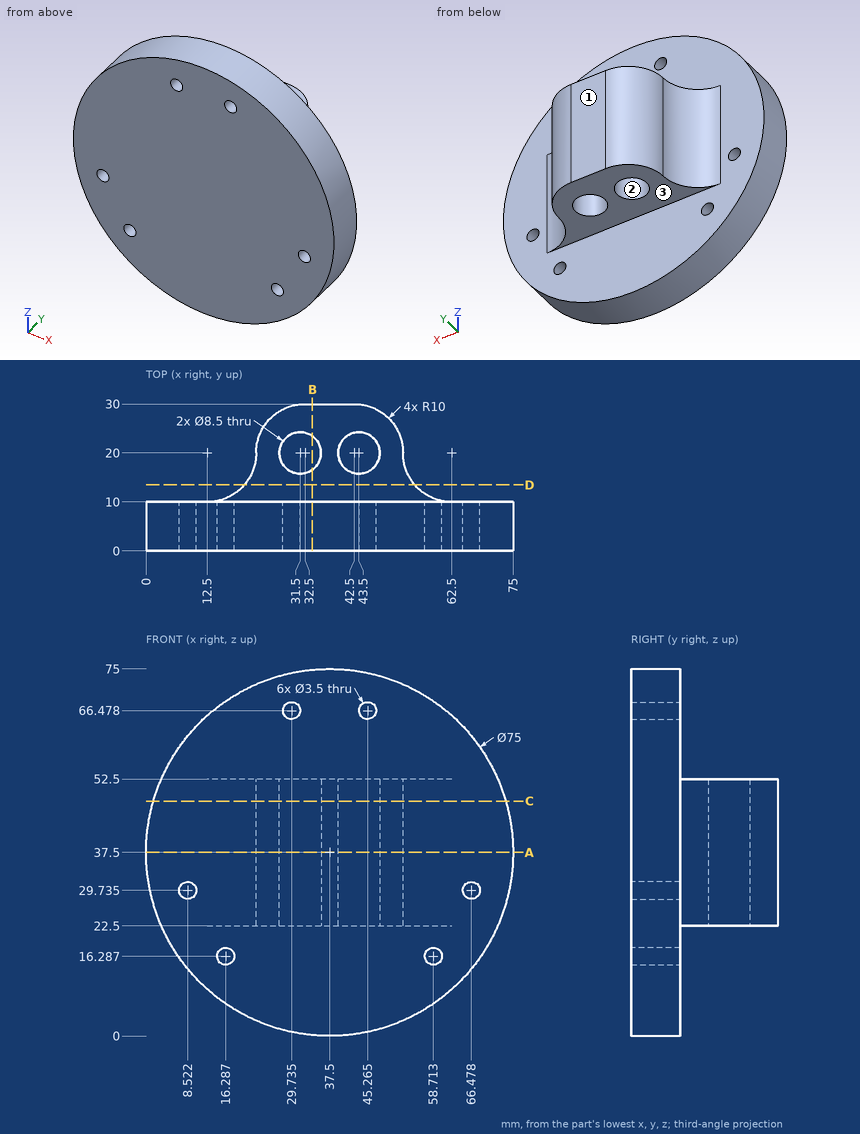
Design review of the part shown in the three views and the two pictorial views. Dimensions are in mm from the part's minimum x, y and z. Give positions to 0.01 mm unless a question says otherwise; leave off trailing zeros. Write each loop counter-clockwise with the first axis right and the second up, starting at its lowest first coordinate (ties: lowest second). Pieces come first, ordered by that corner, then holes. Notation, with made-up numbers: M 10.25,31 L 42.25,31 A28 cw 42.25,50 Z; hole C 27,82.25 d6. An arc over 180 degrees is marked long. Answer in a Markdown table with one row per item.
Item 1: Add section B-B on x = 34. Give the boundary of the cut face in (y, z).
Check sheet entries:
| item | result |
|---|---|
| outline | M 0,0.16 L 10,0.16 L 10,22.5 L 16.56,22.5 L 16.56,52.5 L 10,52.5 L 10,74.84 L 0,74.84 Z; M 23.44,22.5 L 30,22.5 L 30,52.5 L 23.44,52.5 Z |
Item 2: Add section D-D on y = 13.5. Give the boundary of the cut face in (x, z), plus the area to 3 significant figures.
Check sheet entries:
| item | result |
|---|---|
| outline | M 20.1,22.5 L 54.9,22.5 L 54.9,52.5 L 20.1,52.5 Z |
| area | 1,040 mm2 |
Item 3: Add section A-A on z = 37.5. Give the boundary of the cut face in (x, y).
Check sheet entries:
| item | result |
|---|---|
| outline | M 0,0 L 75,0 L 75,10 L 62.5,10 A10 cw 52.5,20 A10 ccw 42.5,30 L 32.5,30 A10 ccw 22.5,20 A10 cw 12.5,10 L 0,10 Z; hole C 31.5,20 d8.5; hole C 43.5,20 d8.5 |
Item 4: For P1, Ø13.5, axis at x = 31.5, y = 20, coming from the +Z side; P2, Ø3, axis at x = 8, z = 44, coming from the -Y side; P3, Ø4, axis at y = 10, z = 55.5, coming from the +X side (1 decimal); P4, Ø3, axis at x = 63.5, z = 32, coming from the +Y side, all flat-tipped, find the tip position at first contact; note any pin that passes through.
Check sheet entries:
| item | result |
|---|---|
| P1 | z = 52.5 |
| P2 | y = 0 |
| P3 | x = 71.4 |
| P4 | y = 10.01 |
Item 5: Add section C-C on z = 48. Give the boundary of the cut face in (x, y).
Check sheet entries:
| item | result |
|---|---|
| outline | M 1.5,0 L 73.5,0 L 73.5,10 L 62.5,10 A10 cw 52.5,20 A10 ccw 42.5,30 L 32.5,30 A10 ccw 22.5,20 A10 cw 12.5,10 L 1.5,10 Z; hole C 31.5,20 d8.5; hole C 43.5,20 d8.5 |
Item 6: Draft analysis for pull direction Y (two halves, no side actions). For the marked faces 1, 2 and 3, state which applies: +Y half, -Y half, draft (parallel to the pull), parting line (faces both ways), or undercut.
Check sheet entries:
| item | result |
|---|---|
| face 1 | +Y half |
| face 2 | undercut |
| face 3 | draft |
Item 7: For line 1 along X through (y, z) = (20, 37.5); line 2 along Y through (x, z) = (55.5, 68.5); line 3 along Z through (x, y) = (37.5, 13.5), list the stretches that pass through material, from the lowest coordinate up.
Check sheet entries:
| item | result |
|---|---|
| line 1 | 22.5 to 27.25, 35.75 to 39.25, 47.75 to 52.5 |
| line 2 | 0 to 10 |
| line 3 | 22.5 to 52.5 |
